Design review of the part built by this model. Coordinates are the model's own, in mm. A direction names the side the tool comes from. Coordinates: 2 decimals unless noted, no trailing zeros. Loops run counter-clockwise (first coordinate to the right, second up) from the corner with the lowest first, then second, coordinate; pieces in that order, holes last. Notation, with made-up numbers: (-36.75, 5) - (-24.75, 5) arc R3 ccw to (-24.75, 10) - close; hole circle Ø8 at (-8.5, 79.5). An arc over 180 degrees is marked (long way). Return JSON: item names as keys, results as strings. Group by question number.
from build123d import *

# Parameters (mm, degrees)
SALIENTE_EXTRUIR1_DEPTH = 5
SALIENTE_EXTRUIR2_DEPTH = 5


with BuildPart() as part:
    # Croquis1 → Saliente-Extruir1 (new body)
    with BuildSketch(Plane(origin=(0, 0, 0), x_dir=(1, 0, 0), z_dir=(0, 1, 0))):
        with BuildLine():
            Line((-62.245, -41.575), (54.245, -41.575))
            ThreePointArc((54.245, -41.575), (59.901854249, -39.231854249), (62.245, -33.575))
            Line((62.245, -33.575), (62.245, 41.575))
            Line((62.245, 41.575), (-62.245, 41.575))
            Line((-62.245, 41.575), (-62.245, -41.575))
        make_face()
    extrude(amount=SALIENTE_EXTRUIR1_DEPTH)

    # Croquis2 → Saliente-Extruir2 (add)
    with BuildSketch(Plane(origin=(0, 0, 0), x_dir=(1, 0, 0), z_dir=(0, 1, 0))):
        with BuildLine():
            Line((52.245, -31.575), (52.245, 31.575))
            Line((52.245, 31.575), (21.4, 31.575))
            Line((21.4, 31.575), (-62.245, 31.575))
            Line((-62.245, 31.575), (-62.245, 36.575))
            Line((-62.245, 36.575), (57.245, 36.575))
            Line((57.245, 36.575), (57.245, -31.575))
            ThreePointArc((57.245, -31.575), (55.780533906, -35.110533906), (52.245, -36.575))
            Line((52.245, -36.575), (-62.245, -36.575))
            Line((-62.245, -36.575), (-62.245, -31.575))
            Line((-62.245, -31.575), (52.245, -31.575))
        make_face()
    extrude(amount=-SALIENTE_EXTRUIR2_DEPTH)


solid = part.part
Item 1: Add section B-B (x = 49.5). State the section outline as (y, z) points (3 decimals), then the cut area to 3 significant figures.
Item 2: Add section C-C (z = 14.5). State the section outline as (x, y) points (3 decimals).
Item 3: For faces 4 (the face through (59.839, 2.465, 39.294)), 5 (the face through (52.245, -2, 0)), 6 (the face through (-3, -2, -36.575)), 7 (the face through (-4, -2, 36.575)), list the 3-axis set-ups (+Z, -Z, +X, -X, +Y, -Y) from which the entire face can be reached by the end or side of a thin tool; tool diameter is ignored.
Item 4: To check wall thickness, follow line 1 (Z direction, x = 10.5, y = -1) (3 decimals); line 2 (Y direction, x = 31, z = -18); line 3 (X direction, y = -0.5, z = 11) (3 decimals). State the ranges of each line that lie inside material, in increasing order. Write a range as from..to.
Item 5: For P1, Ø6, axis at x = 33.5, z = 4, coming from the -Y side; P2, Ø1.5, axis at y = -2, z = 29, coming from the +X side (3 decimals); P3, Ø4, axis at y = -3.5, z = -13.5, coming from the -X side (3 decimals), all flat-tipped, find the tip position at first contact; note any pin that passes through.
Item 6: Add section A-A (y = -2.75). State the section outline as (x, z) points (3 decimals).
Item 7: Draft analysis for pull direction Z (two halves, no side actions). For faces 1 (the face through (55.82, -2.46, 35.07)), 2 (the face through (-6, 0, 0)), 3 (the face through (57.245, -2, -3)), state which applies: pulls with the +Z half, pulls with the -Z half, needs draft (parallel to the pull), parting line crosses it, or undercut.
Answers below:
{
 "1": {"outline": "(-5, -36.575) - (0, -36.575) - (0, -41.575) - (5, -41.575) - (5, 41.575) - (0, 41.575) - (0, 36.575) - (-5, 36.575) - (-5, 31.575) - (0, 31.575) - (0, -31.575) - (-5, -31.575) - close", "area": "466 mm^2"},
 "2": {"outline": "(-62.245, 0) - (52.245, 0) - (52.245, -5) - (57.245, -5) - (57.245, 0) - (62.245, 0) - (62.245, 5) - (-62.245, 5) - close"},
 "3": {"face 4": "+Z, +X, +Y, -Y", "face 5": "-X, -Y", "face 6": "-Z, +X, -X, -Y", "face 7": "+Z, +X, -X, -Y"},
 "4": {"line 1": "z = -36.575..-31.575, 31.575..36.575", "line 2": "y = 0..5", "line 3": "x = 52.245..57.245"},
 "5": {"P1": "stops at y = 0", "P2": "stops at x = 57.245", "P3": "stops at x = 52.245"},
 "6": {"outline": "(-62.245, -36.575) - (57.245, -36.575) - (57.245, 31.575) arc R5 ccw to (52.245, 36.575) - (-62.245, 36.575) - (-62.245, 31.575) - (52.245, 31.575) - (52.245, -31.575) - (-62.245, -31.575) - close"},
 "7": {"face 1": "pulls with the +Z half", "face 2": "undercut", "face 3": "needs draft"}
}
